Autodesk Inventor part; units mm, degrees
ref_plane "YZ Plane" through (0, 0, 0) normal (1, 0, 0) x (0, 1, 0)
ref_plane "XZ Plane" through (0, 0, 0) normal (0, 1, 0) x (-1, 0, 0)
ref_plane "XY Plane" through (0, 0, 0) normal (0, 0, 1) x (1, 0, 0)
sketch "Эскиз1" plane through (0, 0, 0) normal (0, 0, 1) x (1, 0, 0)
  line L0 (0, 0) -> (20, 0)
  line L1 (20, 0) -> (20, 30)
  line L2 (20, 30) -> (0, 30)
  line L3 (0, 30) -> (0, 0)
  dimension "d0" = 20
  dimension "d1" = 30
revolve "Вращение1" add sketch "Эскиз1" angle 360 about axis through (0, 0, 0) along (1, 0, 0)
sketch "Эскиз2" plane through (0, 0, 0) normal (-1, 0, 0) x (0, 0, 1)
  circle A0 centre (0, 5) radius 2
  point P0 (0, 0)
  dimension "d3" = 4
  dimension "d4" = 5
extrude "Выдавливание1" cut sketch "Эскиз2" against normal blind 20
sketch "Эскиз3" plane through (0, 0, 0) normal (0, 0, 1) x (1, 0, 0)
  line L0 (0, 3) -> (0, 7)
  line L1 (0, -30) -> (0, 30) construction
  line L2 (0, 22) -> (4.5, 22) construction
  line L3 (0, 23.0379) -> (4.5, 24.5)
  line L4 (4.5, 24.5) -> (4.5, 22)
  line L5 (0, 0) -> (20, 0)
  line L6 (20, -30) -> (20, 30) construction
  line L7 (0, 22) -> (0, 23.0379)
  line L8 (0, 74) -> (0, 14) construction
  line L9 (0, 20.9621) -> (4.5, 19.5)
  line L10 (4.5, 19.5) -> (4.5, 22)
  line L11 (0, 22) -> (0, 20.9621)
  dimension "d7" = 4.5
  dimension "d8" = 22
  dimension "d10" = 72
  dimension "d12" = 2.5
revolve "Вращение3" cut sketch "Эскиз3" angle 360 about axis through (0, 0, 0) along (1, 0, 0)
properties part number "711116"
Read the model definition and answer for the solid it produces. Units are mm, in the model's axes. A direction names the side the tool comes from. Round coordinates to 2 decimals unless told otherwise and drop trailing zeros. Order: outer loops, then holes, each group sorted by start corner. A loop starts at its lowest first (then second) coordinate and runs counter-clockwise, first axis right, second up. Notation, with made-up numbers: (75, -36) - (123, -36) arc R14 cw to (123, -13) - close; hole circle Ø9 at (73.5, 3). An arc over 180 degrees is marked (long way). Use one line per item in the form item = value. Start each with the question number.
(1) The part is cut by section D-D (x = 1.5). Give the vertices of the cut face in (y, z).
(2) The part is cut by section B-B (x = 5.25). Give the vertices of the cut face in (y, z).
(3) Determine the mould class of faces 3 (the face through (9.86, -29.97, -1.32)), 4 (the face through (4.5, -16.45, -10.77)), 5 (the face through (0, 9, -22)) for opening direction Y: +Y half, -Y half, draft (parallel to the pull), parting line (faces both ways), or undercut.
(4) The part is cut by section A-A (z = 0). Give the vertices of the cut face in (x, y).
(5) The part is cut by section C-C (y = 0). Give the vertices of the cut face in (x, z), then the cut area to 3 significant figures.
(6) For faces 1 (the face through (0, 0, 0)), 2 (the face through (0.28, -5.01, -22.58)), determine the directions among +Z, -Z, +X, -X, +Y, -Y from which every point of the face is accessible in a straight line to the end or side of a thin tool.
(7) Flat-ended cylindrical pins translate along their axes: pin 1 Ø2 at (x, y) = (11.5, 19) entering from +Z; pin 2 Ø1 at (y, z) = (11.5, 19) entering from -X; pin 3 Ø1 at (x, y) = (9.5, 6.5) entering from -Z. Find the tip coordinate at first contact, or state that the pin passes through.
(8) Find the intervals of material crossed by line 1 along Z through (x, y) = (1.75, 6); line 2 along Z through (x, y) = (4, -14); line 3 along Y through (x, z) = (2.75, -4), in increasing order. Write a range as from..to.
Checked values:
q1.outline = circle Ø60 at (0, 0); circle Ø40.95 at (0, 0); hole circle Ø47.05 at (0, 0); hole circle Ø4 at (5, 0)
q2.outline = circle Ø60 at (0, 0); hole circle Ø4 at (5, 0)
q3.face_3 = parting line
q3.face_4 = undercut
q3.face_5 = draft
q4.outline = (0, -30) - (20, -30) - (20, 3) - (0, 3) - (0, -20.96) - (4.5, -19.5) - (4.5, -24.5) - (0, -23.04) - close; (0, 7) - (20, 7) - (20, 30) - (0, 30) - (0, 23.04) - (4.5, 24.5) - (4.5, 19.5) - (0, 20.96) - close
q5.outline = (0, -30) - (20, -30) - (20, 30) - (0, 30) - (0, 23.04) - (4.5, 24.5) - (4.5, 19.5) - (0, 20.96) - (0, -20.96) - (4.5, -19.5) - (4.5, -24.5) - (0, -23.04) - close
q5.area = 1,170 mm^2
q6.face_1 = +Z, -Z, -X, +Y, -Y
q6.face_2 = none
q7.pin_1 = 24
q7.pin_2 = 4.5
q7.pin_3 = -29.39
q8.line_1 = -29.39..-22.83, -19.49..-1.73, 1.73..19.49, 22.83..29.39
q8.line_2 = -26.53..-19.91, -13.81..13.81, 19.91..26.53
q8.line_3 = -29.73..-23.59, -19.67..19.67, 23.59..29.73
